Work out the finished part from the listing and answer in its coordinate system (mm). Face numbers are marked on the shaded views. A direction names the side the tool comes from. Round coordinates to 2 decimals unless told otherwise and drop trailing zeros. Loops run counter-clockwise (first coordinate to the right, second up) from the corner with the lowest first, then second, coordinate; pieces in that order, holes last.
```python
from build123d import *

# Parameters (mm, degrees)
F1_DEPTH = 159
F2_W     = 22
F2_H     = 37
F3_DEPTH = 45.8205918838
F4_W     = 40
F4_H     = 9.5769511967
F5_DEPTH = 65.001
F6_R     = 5


with BuildPart() as f1:
    # F0 (on Front) → F1 (new body)
    with BuildSketch(Plane.XZ):
        with BuildLine():
            ThreePointArc((0.6666666667, 1.8856180832), (2, 0), (0.6666666667, -1.8856180832))
            ThreePointArc((0.6666666667, -1.8856180832), (-0.5412414523, -2.7992650141), (-1, -4.2426406871))
            Line((-1, -4.2426406871), (-1, -13.8195918838))
            Line((-1, -13.8195918838), (0, -13.8195918838))
            Line((0, -13.8195918838), (0, -4.2426406871))
            ThreePointArc((0, -4.2426406871), (0.2752551286, -3.3766152833), (1, -2.8284271247))
            ThreePointArc((1, -2.8284271247), (3, 0), (1, 2.8284271247))
            ThreePointArc((1, 2.8284271247), (0.2752551286, 3.3766152833), (0, 4.2426406871))
            Line((0, 4.2426406871), (0, 29.5))
            ThreePointArc((0, 29.5), (0.4393398282, 30.5606601718), (1.5, 31))
            Line((1.5, 31), (61.5, 31))
            ThreePointArc((61.5, 31), (62.5606601718, 30.5606601718), (63, 29.5))
            Line((63, 29.5), (63, 4.2426406871))
            ThreePointArc((63, 4.2426406871), (62.7247448714, 3.3766152833), (62, 2.8284271247))
            ThreePointArc((62, 2.8284271247), (60, 0), (62, -2.8284271247))
            ThreePointArc((62, -2.8284271247), (62.7247448714, -3.3766152833), (63, -4.2426406871))
            Line((63, -4.2426406871), (63, -13.8195918838))
            Line((63, -13.8195918838), (64, -13.8195918838))
            Line((64, -13.8195918838), (64, -4.2426406871))
            ThreePointArc((64, -4.2426406871), (63.5412414523, -2.7992650141), (62.3333333333, -1.8856180832))
            ThreePointArc((62.3333333333, -1.8856180832), (61, 0), (62.3333333333, 1.8856180832))
            ThreePointArc((62.3333333333, 1.8856180832), (63.5412414523, 2.7992650141), (64, 4.2426406871))
            Line((64, 4.2426406871), (64, 29.5))
            ThreePointArc((64, 29.5), (63.267766953, 31.267766953), (61.5, 32))
            Line((61.5, 32), (1.5, 32))
            ThreePointArc((1.5, 32), (-0.267766953, 31.267766953), (-1, 29.5))
            Line((-1, 29.5), (-1, 4.2426406871))
            ThreePointArc((-1, 4.2426406871), (-0.5412414523, 2.7992650141), (0.6666666667, 1.8856180832))
        make_face()
    extrude(amount=F1_DEPTH)

    # F2 (on face) → F3 (cut, through all)
    with BuildSketch(Plane.XY.offset(32)):
        with Locations((31.5, -118)):
            Rectangle(F2_W, F2_H)
        with Locations((31.5, -41)):
            Rectangle(F2_W, F2_H)
    extrude(amount=-F3_DEPTH, mode=Mode.SUBTRACT)

    # F4 (on face) → F5 (cut, through all)
    with BuildSketch(Plane.YZ.offset(64)):
        with BuildLine():
            Line((-99.5, -4.2426406871), (-59.5, -4.2426406871))
            Line((-59.5, -4.2426406871), (-59.5, 6.1804081162))
            ThreePointArc((-59.5, 6.1804081162), (-60.9644660941, 9.7159420222), (-64.5, 11.1804081162))
            Line((-64.5, 11.1804081162), (-94.5, 11.1804081162))
            ThreePointArc((-94.5, 11.1804081162), (-98.0355339059, 9.7159420222), (-99.5, 6.1804081162))
            Line((-99.5, 6.1804081162), (-99.5, -4.2426406871))
        make_face()
        with Locations((-79.5, -9.0311162854)):
            Rectangle(F4_W, F4_H)
    extrude(amount=-F5_DEPTH, mode=Mode.SUBTRACT)

    # F6
    f6_edges = [f1.edges().sort_by_distance(p)[0] for p in [
        (63.5, 0, -13.819592),
        (63.5, -99.5, -13.819592),
        (63.5, -59.5, -13.819592),
        (-0.5, -99.5, -13.819592),
        (-0.5, -59.5, -13.819592),
    ]]
    fillet(f6_edges, radius=F6_R)


solid = f1.part
```
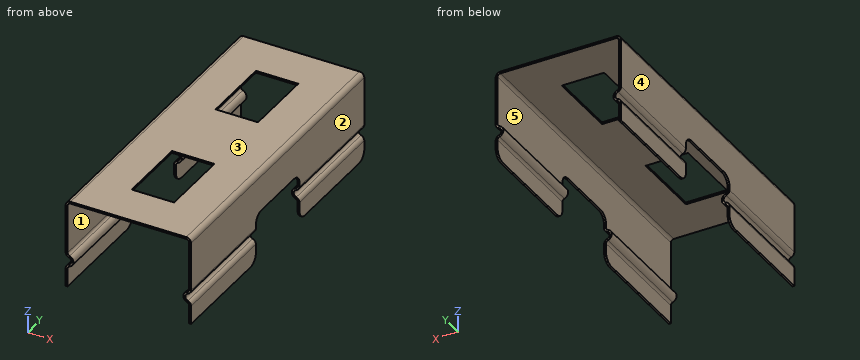
1. Find section C-C (x = 29.5). Write down the section's boundary in (y, z), then the cut area to 3 significant figures.
Answer key:
outline: (-159, 31) - (-136.5, 31) - (-136.5, 32) - (-159, 32) - close; (-99.5, 31) - (-59.5, 31) - (-59.5, 32) - (-99.5, 32) - close; (-22.5, 31) - (0, 31) - (0, 32) - (-22.5, 32) - close
area: 85.0 mm2
2. Given pin 1 (0.5 mm diameter, centred on y = -33.5, z = 31.5, fed in from -X); pin 2 (4 mm diameter, centred on x = 40.5, y = -84.5, fed in from -Z); pin 3 (0.8 mm diameter, centred on x = 30.5, z = 31.5, fed in from +Y); pin 4 (8 mm diameter, centred on y = -85.5, z = 5, fed in from +X), each flat-ended and moving along its own axis, determine where each tip first touches the part or whether it passes through.
Answer key:
pin 1: stops at x = -0.29
pin 2: stops at z = 31
pin 3: stops at y = 0
pin 4: passes through
3. Find section D-D (z = 8). Write down the section's boundary in (x, y), then the cut area to 3 significant figures.
Answer key:
outline: (-1, -159) - (0, -159) - (0, -99.16) - (-1, -99.16) - close; (-1, -59.84) - (0, -59.84) - (0, 0) - (-1, 0) - close; (63, -159) - (64, -159) - (64, -99.16) - (63, -99.16) - close; (63, -59.84) - (64, -59.84) - (64, 0) - (63, 0) - close
area: 239 mm2
4. Find section A-A (z = 28). Write down the section's boundary in (x, y), then the cut area to 3 significant figures.
Answer key:
outline: (-1, -159) - (0, -159) - (0, 0) - (-1, 0) - close; (63, -159) - (64, -159) - (64, 0) - (63, 0) - close
area: 318 mm2
5. Which of the six approach directions +Z, -Z, +X, -X, +Y, -Y give full straight-line access (tool end or side, diameter ignored) to the marked faces 1 and 2?
Answer key:
face 1: +Y, -Y
face 2: +Z, -Z, +X, +Y, -Y
6. Consider probe 1 along X at (y, z) = (-49.5, 23); probe 2 along Z at (x, y) = (55, -43); probe 3 along X at (y, z) = (-152, -2). Determine where each line is inside the solid, lowest interval first.
Answer key:
probe 1: x = -1 to 0, 63 to 64
probe 2: z = 31 to 32
probe 3: x = 0.4 to 2.24, 60.76 to 62.6
7. Determine the mould class of the marked faces 3, 4 and 5 for opening direction X: +X half, -X half, draft (parallel to the pull), parting line (faces both ways), or undercut.
Answer key:
face 3: draft
face 4: -X half
face 5: undercut
